Here's the drawing with two shaded views (mm, measured from the low corner). I have some questions. Round coordinates to 2 decimals unless told otherwise and drop trailing zeros. Order: outer loops, then holes, each group sorted by start corner. A loop starts at its lowest first (then second) coordinate and runs counter-clockwise, first axis right, second up. Notation, with made-up numbers: (70, 60.5) -> (86, 60.5) arc R16 ccw to (86, 89.5) -> close; hole circle Ø7 at (40, 29.25). An arc over 180 degrees is marked (long way). Use a Markdown table: item, result. Add a question column.
Q1. I need wall thicknesses on line 1 along X through (y, z) = (1.15, 2); line 2 along X through (y, z) = (1.1, 2.55); line 3 along Z through (x, y) = (2, 2). Which ranges of each line are inside material? Lowest first, please. Write a range as [from, to].
Q2. If we section it at C-C on x = 41.5: List the corners of the cut face in (y, z) for me.
Q3. If we section it at B-B on z = 1.5: List the corners of the cut face in (x, y) for me.
Q4. If we section it at A-A on y = 2.1: List the corners of the cut face in (x, z) for me.
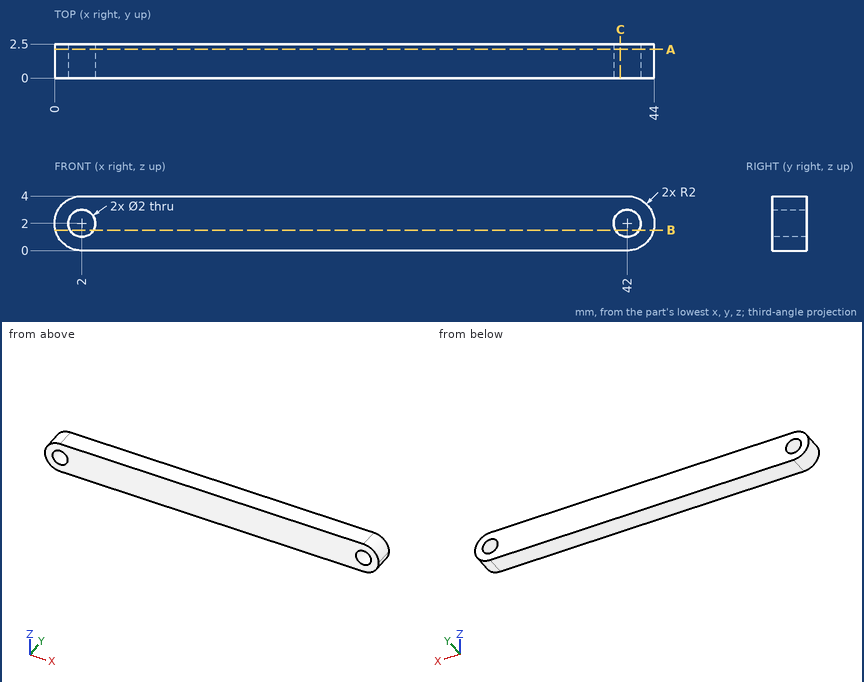
Answer below:
| question | item | result |
|---|---|---|
| 1 | line 1 | [0, 1], [3, 41], [43, 44] |
| 1 | line 2 | [0.08, 1.16], [2.84, 41.16], [42.84, 43.92] |
| 1 | line 3 | [0, 1], [3, 4] |
| 2 | outline | (0, 0) -> (2.5, 0) -> (2.5, 1.13) -> (0, 1.13) -> close; (0, 2.87) -> (2.5, 2.87) -> (2.5, 4) -> (0, 4) -> close |
| 3 | outline | (0.06, 0) -> (1.13, 0) -> (1.13, 2.5) -> (0.06, 2.5) -> close; (2.87, 0) -> (41.13, 0) -> (41.13, 2.5) -> (2.87, 2.5) -> close; (42.87, 0) -> (43.94, 0) -> (43.94, 2.5) -> (42.87, 2.5) -> close |
| 4 | outline | (2, 0) -> (42, 0) arc R2 ccw to (42, 4) -> (2, 4) arc R2 ccw to start; hole circle Ø2 at (2, 2); hole circle Ø2 at (42, 2) |
